Input: part model. Units: mm. Frame: model coordinates. A direction names the side the tool comes from. Give positions to 0.01 mm unless a question says otherwise; leave off trailing zeros. Order: outer loops, then holes, each group sorted by start corner. A loop starts at its lowest first (then second) coordinate and runs counter-clockwise, first axis right, second up. Notation, with made-up numbers: (-10, 44) - (42, 44) arc R23 ccw to (42, 67) - close; hole circle Ø7 at (21.25, 57.5). An arc over 180 degrees is marked (long way). Use a Markdown table: item, result.
Autodesk Inventor part; units mm, degrees
ref_plane "YZ Plane" through (0, 0, 0) normal (1, 0, 0) x (0, 1, 0)
ref_plane "XZ Plane" through (0, 0, 0) normal (0, 1, 0) x (-1, 0, 0)
ref_plane "XY Plane" through (0, 0, 0) normal (0, 0, 1) x (1, 0, 0)
sketch "Sketch1" plane through (0, 0, 0) normal (1, 0, 0) x (0, 1, 0)
  line L0 (0, 0) -> (40, 0)
  line L1 (40, 0) -> (40, -50)
  line L2 (0, 0) -> (10, 0)
  line L3 (10, -50) -> (0, -50)
  line L4 (0, -50) -> (0, 0)
  line L5 (40, -50) -> (40, -280)
  line L6 (40, -280) -> (0, -280)
  line L7 (0, -280) -> (0, -230)
  line L8 (0, -230) -> (10, -230)
  line L9 (10, -230) -> (10, -50)
  dimension "d0" = 40
  dimension "d1" = 50
  dimension "d3" = 230
  dimension "d4" = 50
  dimension "d5" = 10
extrude "Extrusion1" add sketch "Sketch1" along normal blind 5
properties part number "cover"
1. Pin query (flat end, axial travel): pin 1 (2.5 mm diameter, centred on x = 2.5, z = -113.5, fed in from -Y). Return the tip coordinate at first contact, or that it passes through.
Response:
| item | result |
|---|---|
| pin 1 | stops at y = 10 |
2. Section query A-A (y = 5.5). Return loops of the section in (x, z), then the cut area to 3 significant figures.
Response:
| item | result |
|---|---|
| outline | (0, -280) - (5, -280) - (5, -230) - (0, -230) - close; (0, -50) - (5, -50) - (5, 0) - (0, 0) - close |
| area | 500 mm^2 |
3. Section query C-C (z = -210.5). Return loops of the section in (x, y).
Response:
| item | result |
|---|---|
| outline | (0, 10) - (5, 10) - (5, 40) - (0, 40) - close |
4. Material intervals for line 1 along Z through (x, y) = (4.3, 2.5); line 2 along Y through (x, z) = (2.3, -92), sorted ascending.
Response:
| item | result |
|---|---|
| line 1 | z = -280 to -230, -50 to 0 |
| line 2 | y = 10 to 40 |
5. Mould query, pull axis Z, two halves, no side actions, for faces 3 (the face through (2, 5, -230)), 4 (the face through (5, 20, -138)), 5 (the face through (2, 20, 0)). Classes: pulls with the +Z half, pulls with the -Z half, needs draft (parallel to the pull), parting line crosses it, or undercut.
Response:
| item | result |
|---|---|
| face 3 | undercut |
| face 4 | needs draft |
| face 5 | pulls with the +Z half |
6. Section query B-B (x = 3.85). Return loops of the section in (y, z).
Response:
| item | result |
|---|---|
| outline | (0, -280) - (40, -280) - (40, 0) - (0, 0) - (0, -50) - (10, -50) - (10, -230) - (0, -230) - close |
7. Set-up query: faces 1 (the face through (2, 0, -25)), 2 (the face through (2, 10, -141)). Return all of +Z, -Z, +X, -X, +Y, -Y with unobstructed straight access to the full face (end or side cutting, diameter ignored); none if empty.
Response:
| item | result |
|---|---|
| face 1 | +Z, -Z, +X, -X, -Y |
| face 2 | +X, -X, -Y |
